```python
from build123d import *

# Parameters (mm, degrees)
SKETCH1_R           = 25.275
SKETCH1_R_2         = 20.625
BOSS_EXTRUDE1_DEPTH = 45
SKETCH2_R           = 22.625
CUT_EXTRUDE1_DEPTH  = 3.5
SKETCH3_R           = 23.625
CUT_EXTRUDE2_DEPTH  = 1
SKETCH4_R           = 0.5
CUT_EXTRUDE3_DEPTH  = 47.5


with BuildPart() as part:
    # Sketch1 → Boss-Extrude1 (new body)
    with BuildSketch(Plane(origin=(0, 0, 0), x_dir=(1, 0, 0), z_dir=(0, 1, 0))):
        Circle(SKETCH1_R)
        Circle(SKETCH1_R_2, mode=Mode.SUBTRACT)
    extrude(amount=BOSS_EXTRUDE1_DEPTH)

    # Sketch2 → Cut-Extrude1 (cut)
    with BuildSketch(Plane.XZ):
        Circle(SKETCH2_R)
    extrude(amount=-CUT_EXTRUDE1_DEPTH, mode=Mode.SUBTRACT)

    # Sketch3 → Cut-Extrude2 (cut)
    with BuildSketch(Plane(origin=(0, 45, 0), x_dir=(1, 0, 0), z_dir=(0, 1, 0))):
        Circle(SKETCH3_R)
    extrude(amount=-CUT_EXTRUDE2_DEPTH, mode=Mode.SUBTRACT)

    # Sketch4 → Cut-Extrude3 (cut)
    with BuildSketch(Plane(origin=(0, 45, 0), x_dir=(1, 0, 0), z_dir=(0, 1, 0))):
        with Locations((0, 23.625)):
            Circle(SKETCH4_R)
    extrude(amount=-CUT_EXTRUDE3_DEPTH, mode=Mode.SUBTRACT)


solid = part.part
```
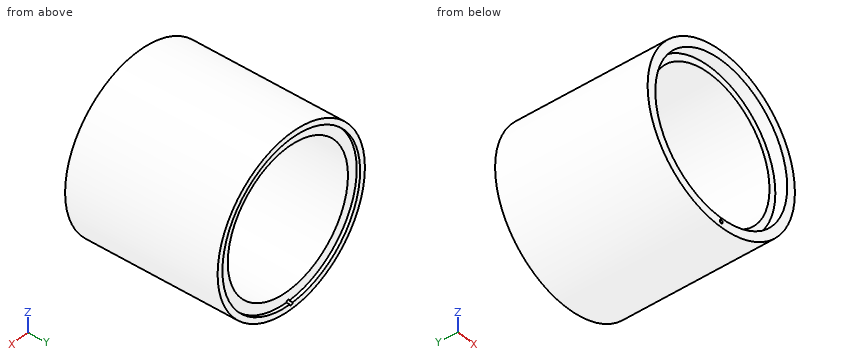
CAD build for the part. Positions are in the model's coordinates, mm. Give positions to 0.01 mm unless a question says otherwise; leave off trailing zeros. Order: outer loops, then holes, each group sorted by start corner. A loop starts at its lowest first (then second) coordinate and runs counter-clockwise, first axis right, second up.
(1) Saw through at C-C, the plane y = 17. Give the cut face in (x, z) (3 decimals).
(2) Saw through at A-A, the plane z = -16. Give the cut face in (x, y).
(3) Drill centre lines: L1, parallel to Z at x = 0, y = 2.3 (3 decimals); L2, parallel to Z at x = 0, y = 16.5 (3 decimals); L3, parallel to X at y = 18, z = 17.5. Where is each one in solid material? Low to high.
(4) Flat gauge pins, fed straight in: pin 1 (3 mm diameter, centred on x = 17, y = 30, fed in from -Z); pin 2 (8 mm diameter, centred on y = 11.5, z = 15, fed in from -X); pin 3 (12 mm diameter, centred on y = 32, z = 12, fed in from +X). Where does each tip first touch, or does it go through?
(5) Saw through at B-B, the plane x = 18.5. Give the cut face in (y, z), then the cut area to 3 significant figures.
Results found:
1. outline: circle Ø50.55 at (0, 0); hole circle Ø41.25 at (0, 0); hole circle Ø1 at (0, -23.625)
2. outline: (-19.57, 0) - (-16, 0) - (-16, 3.5) - (-13.02, 3.5) - (-13.02, 44) - (-17.38, 44) - (-17.38, 45) - (-19.57, 45) - close; (13.02, 3.5) - (16, 3.5) - (16, 0) - (19.57, 0) - (19.57, 45) - (17.38, 45) - (17.38, 44) - (13.02, 44) - close
3. L1: z = -25.275 to -24.125, -23.125 to -22.625, 22.625 to 25.275
3. L2: z = -25.275 to -24.125, -23.125 to -20.625, 20.625 to 25.275
3. L3: x = -18.24 to -10.92, 10.92 to 18.24
4. pin 1: stops at z = -19.96
4. pin 2: stops at x = -22.76
4. pin 3: stops at x = 24.55
5. outline: (0, -17.22) - (45, -17.22) - (45, -14.69) - (44, -14.69) - (44, -9.12) - (3.5, -9.12) - (3.5, -13.02) - (0, -13.02) - close; (0, 13.02) - (3.5, 13.02) - (3.5, 9.12) - (44, 9.12) - (44, 14.69) - (45, 14.69) - (45, 17.22) - (0, 17.22) - close
5. area: 691 mm2
